CAD build for the part. Positions are in the model's coordinates, mm. Coordinates: 2 decimals unless noted, no trailing zeros. Write each loop counter-clockwise with the first axis right and the second up, starting at its lowest first coordinate (ties: lowest second). Pieces come first, ordered by that corner, then holes. Notation, with made-up numbers: (75.25, 14) - (85.25, 14) arc R22 ccw to (85.25, 45) - close; hole circle Ø6 at (64.5, -18.75). An arc over 180 degrees is marked (long way). Answer in a Markdown table with one row per item. Add a question column.
Q1. Band-saw the part on A-A (x = 14.25). List the corners of the cut face in (y, z), and give its area (3 significant figures).
Q2. Pin check, flat tips, straight feed: pin 1 (4 mm diameter, centred on x = 10, z = -55, fed in from -Y); pin 2 (5 mm diameter, centred on x = 16.5, y = 19, fed in from +Z); pin 3 (4 mm diameter, centred on x = 20, z = 45.5, fed in from -Y). Stop position of each tip, or through.
Q3. Band-saw the part on C-C (z = -83.5). List the corners of the cut face in (x, y).
Q4. Band-saw the part on B-B (y = 19). List the corners of the cut face in (x, z), and give its area (3 significant figures).
Q5. Drill centre lines: line 1 along Y through (x, z) = (13, -41.5); line 2 along Z through (x, y) = (4.5, 12); line 3 along Z through (x, y) = (16.75, -48.5). Where is each one in solid material? Low to high. Write a range as from..to.
```python
from build123d import *

# Parameters (mm, degrees)
F1_DEPTH = 25.4


# Not quite as in the source:
# - the program builds the solid bodies; features that only make, move or delete a surface that nothing else refers to are left out


with BuildPart() as f1:
    # F0 (on Right) → F1 (new body)
    with BuildSketch(Plane.YZ):
        with BuildLine():
            Line((30.5899139494, 31.8673923612), (-13.4478956461, 64.2119422555))
            Line((-13.4478956461, 64.2119422555), (-50.8971004581, 64.2119422555))
            Line((-50.8971004581, 64.2119422555), (-68.4238471531, -47.566784402))
            ThreePointArc((-68.4238471531, -47.566784402), (-66.9375558311, -52.7225543163), (-62.0332139244, -54.8993537478))
            Line((-62.0332139244, -54.8993537478), (17.1407288117, -53.4367848312))
            ThreePointArc((17.1407288117, -53.4367848312), (21.6644422357, -55.21340817), (23.6069282635, -59.6684190188))
            Line((23.6069282635, -59.6684190188), (24.2505592335, -94.5104021757))
            Line((24.2505592335, -94.5104021757), (30.5899139494, -94.5104021757))
            Line((30.5899139494, -94.5104021757), (30.5899139494, 31.8673923612))
        make_face()
    extrude(amount=F1_DEPTH)


solid = f1.part
```
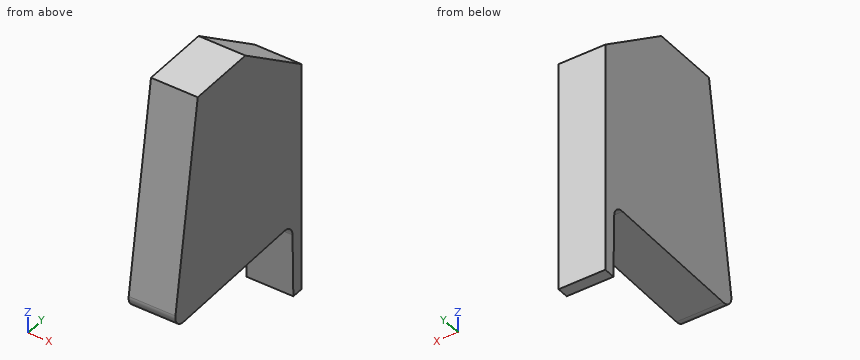
Checked values:
| question | item | result |
|---|---|---|
| 1 | outline | (-68.42, -47.57) arc R6.35 ccw to (-62.03, -54.9) - (17.14, -53.44) arc R6.35 cw to (23.61, -59.67) - (24.25, -94.51) - (30.59, -94.51) - (30.59, 31.87) - (-13.45, 64.21) - (-50.9, 64.21) - close |
| 1 | area | 10,300 mm² |
| 2 | pin 1 | stops at y = -66.68 |
| 2 | pin 2 | stops at z = 42.22 |
| 2 | pin 3 | stops at y = -54.14 |
| 3 | outline | (0, 24.05) - (25.4, 24.05) - (25.4, 30.59) - (0, 30.59) - close |
| 4 | outline | (0, -53.68) - (25.4, -53.68) - (25.4, 40.38) - (0, 40.38) - close |
| 4 | area | 2,390 mm² |
| 5 | line 1 | y = -67.47..30.59 |
| 5 | line 2 | z = -53.53..45.52 |
| 5 | line 3 | z = -54.65..64.21 |
